```python
from build123d import *

# Parameters (mm, degrees)
F0_R     = 4.025
F1_DEPTH = 13
F2_R     = 4.05
F3_DEPTH = 200
F5_DEPTH = 25
F6_R     = 5
F6_R_2   = 3.975
F7_DEPTH = 1
F8_DEPTH = 8


with BuildPart() as f1:
    # F0 (on Top) → F1 (new body)
    with BuildSketch(Plane.XY):
        with BuildLine():
            Line((38, 0), (0, 0))
            Line((0, 0), (-38, 0))
            ThreePointArc((-38, 0), (-44.5, 6.5), (-51, 0))
            Line((-51, 0), (-51, -37.5))
            Line((-51, -37.5), (0, -37.5))
            Line((0, -37.5), (51, -37.5))
            Line((51, -37.5), (51, 0))
            ThreePointArc((51, 0), (44.5, 6.5), (38, 0))
        make_face()
        with Locations((-44.5, 0)):
            Circle(F0_R, mode=Mode.SUBTRACT)
        with Locations((44.5, 0)):
            Circle(F0_R, mode=Mode.SUBTRACT)
    extrude(amount=F1_DEPTH)

    # F2 (on face) → F3 (cut)
    with BuildSketch(Plane.YZ.offset(51)):
        with Locations((-10, 6.5)):
            Circle(F2_R)
        with Locations((-31, 6.5)):
            Circle(F2_R)
    extrude(amount=-F3_DEPTH, mode=Mode.SUBTRACT)

    # F4 (on face) → F5 (cut)
    with BuildSketch(Plane.XY.offset(13)):
        Polygon((-23, -30.980762), (-8, -5), (-38, -5), align=None)
        Polygon((15, -30.980762), (0, -5), (-15, -30.980762), align=None)
        Polygon((23, -30.980762), (38, -5), (8, -5), align=None)
    extrude(amount=-F5_DEPTH, mode=Mode.SUBTRACT)

    # F6 (on face) → F7 (join)
    with BuildSketch(Plane(origin=(0, 0, 0), x_dir=(-1, 0, 0), z_dir=(0, 1, 0))):
        with Locations((0, 6.5)):
            Circle(F6_R)
        with Locations((0, 6.445146)):
            Circle(F6_R_2, mode=Mode.SUBTRACT)
    extrude(amount=F7_DEPTH)

    # F6 (on face) → F8 (join)
    with BuildSketch(Plane(origin=(0, 0, 0), x_dir=(-1, 0, 0), z_dir=(0, 1, 0))):
        with Locations((0, 6.445146)):
            Circle(F6_R_2)
    extrude(amount=F8_DEPTH)


solid = f1.part
```
Build history of the part. All positions in model axes, mm. A direction names the side the tool comes from. Round coordinates to 2 decimals unless told otherwise and drop trailing zeros. Write each loop counter-clockwise with the first axis right and the second up, starting at its lowest first coordinate (ties: lowest second). Pieces come first, ordered by that corner, then holes. Notation, with made-up numbers: (16.5, 50) - (41.5, 50) arc R22 cw to (41.5, 87) - close; hole circle Ø7 at (43, 6). An arc over 180 degrees is marked (long way). Write each question's results on one line, items separated by ' | '. Start each with the question number.
Item 1: Saw through at A-A (x = -44.5). Write the cut outline in (y, z) (3 decimals).
Item 2: Which spindle directions (+Z, -Z, +X, -X, +Y, -Y) get a long thin tool onto all of the face, cutting with end or side? Do faces 4 (the face through (-1, -37.5, 6)), 5 (the face through (-23, -5, 7)), 6 (the face through (0, 1, 2)). Say none if no direction does.
Item 3: Saw through at C-C (x = 10). Write the cut outline in (y, z), and give its area (3 significant figures).
Item 4: Mould opens along X. For faces 1 (the face through (51, -19, 6)), 2 (the face through (-6.846, -13.214, 4.036)), 3 (the face through (44.6, 6.5, 6.4)) say: pulls with the +X half, pulls with the -X half, needs draft (parallel to the pull), parting line crosses it, or undercut.
Item 5: Wall check: L1, parallel to Z at x = 45, y = -10; L2, parallel to Y at x = 46, z = 4; L3, parallel to X at y = -18, z = 5.25. Give the ranges that are in metal, low to high. Write a range as [from, to].
Item 6: Saw through at B-B (y = -22). Write the cut outline in (x, z).
Item 7: Saw through at D-D (y = -13). State how many separate pieces and enclosed holes the cut face has, and give its area (3 significant figures).
Item 8: Drop flat-ended pins along their axis: P1, Ø5, axis at x = -5.5, z = 11, coming from the +Y side; P2, Ø1.2, axis at x = 6.5, z = 12, coming from the +Y side. Give the stop position or say it passes through.
Results are:
1) outline: (-37.5, 0) - (-4.025, 0) - (-4.025, 13) - (-37.5, 13) - close; (4.025, 0) - (6.5, 0) - (6.5, 13) - (4.025, 13) - close; hole circle Ø8.1 at (-31, 6.5); hole circle Ø8.1 at (-10, 6.5)
2) face 4: +Z, -Z, +X, -X, -Y | face 5: +Z, -Z | face 6: +Y
3) outline: (-37.5, 0) - (-30.98, 0) - (-30.98, 2.45) arc R4.05 cw (long way) to (-30.98, 10.55) - (-30.98, 13) - (-37.5, 13) - close; (-22.32, 0) - (-8.46, 0) - (-8.46, 2.75) arc R4.05 cw (long way) to (-8.46, 10.25) - (-8.46, 13) - (-22.32, 13) - close; (-5, 0) - (0, 0) - (0, 13) - (-5, 13) - close | area: 266 mm²
4) face 1: pulls with the +X half | face 2: needs draft | face 3: undercut
5) L1: z = [0, 2.45], [10.55, 13] | L2: y = [-37.5, -34.19], [-27.81, -13.19], [-6.81, -3.74], [3.74, 6.32] | L3: x = [-51, -30.49], [-15.51, -7.51], [7.51, 15.51], [30.49, 51]
6) outline: (-51, 0) - (-28.19, 0) - (-28.19, 13) - (-51, 13) - close; (-17.81, 0) - (-9.81, 0) - (-9.81, 13) - (-17.81, 13) - close; (9.81, 0) - (17.81, 0) - (17.81, 13) - (9.81, 13) - close; (28.19, 0) - (51, 0) - (51, 13) - (28.19, 13) - close
7) separate pieces: 8 | enclosed holes: 0 | area: 387 mm²
8) P1: stops at y = 1 | P2: stops at y = 0
